```python
from build123d import *

# Parameters (mm, degrees)
SKETCH1_R                                 = 44.5
BOSS_EXTRUDE1_DEPTH                       = 24.13
SHELL1_T                                  = -5
CSK_FOR_0_FLAT_HEAD_MACHINE_SCREW_2_COUNT = 2
CSK_FOR_0_FLAT_HEAD_MACHINE_SCREW_2_PITCH = 69.412105808
CIRPATTERN1_COUNT                         = 8
FILLET1_R                                 = 10


with BuildPart() as part:
    # Sketch1 → Boss-Extrude1 (new, symmetric)
    with BuildSketch(Plane.XY):
        with Locations(Location((0, 0, 0), (0, 0, 180))):
            Circle(SKETCH1_R)
    extrude(amount=BOSS_EXTRUDE1_DEPTH, both=True)

    # Shell1
    shell1_openings = [part.faces().sort_by_distance(p)[0] for p in [
        (0, 0, 24.13),
    ]]
    offset(amount=SHELL1_T, openings=shell1_openings, kind=Kind.INTERSECTION)

    # Sketch5 → CSK for #0 Flat Head Machine Screw (100)1 (revolve, cut)
    with BuildSketch(Plane(origin=(-1.269301035, 41.980815558, 24.13), x_dir=(0, -1, 0), z_dir=(1, 0, 0))):
        Polygon((0, 0), (0, 3.07416509), (0.889, 2.54), (0.889, 0.5221717), (1.5113, 0), align=None)
    csk_for_0_flat_head_machine_screw_100 = revolve(axis=Axis((-1.269301035, 41.980815558, 30.48), (0, 0, -1)), mode=Mode.SUBTRACT)

    # CSK for _0 Flat Head Machine Screw _ 2: CSK for #0 Flat Head Machine Screw (100)1 ×2
    with Locations(*[Vector(0.9567328467758284, -0.2909677987341887, 0) * (i * CSK_FOR_0_FLAT_HEAD_MACHINE_SCREW_2_PITCH) for i in range(1, CSK_FOR_0_FLAT_HEAD_MACHINE_SCREW_2_COUNT)]):
        add(csk_for_0_flat_head_machine_screw_100, mode=Mode.SUBTRACT)

    # CirPattern1: CSK for #0 Flat Head Machine Screw (100)1 ×8 about axis
    cirpattern1_axis = Axis((0, 0, 0), (0, 0, 1))
    for i in range(1, CIRPATTERN1_COUNT):
        add(csk_for_0_flat_head_machine_screw_100.rotate(cirpattern1_axis, i * 360 / CIRPATTERN1_COUNT), mode=Mode.SUBTRACT)

    # CirPattern1 copy 1 sketch → CirPattern1 copy 1 (revolve, cut)
    with BuildSketch(Plane(origin=(30.656906272, 61.464315428, 24.13), x_dir=(0.7071067811865475, -0.7071067811865476, 0), z_dir=(0.7071067811865476, 0.7071067811865475, 0))):
        Polygon((0, 0), (0, 3.07416509), (0.889, 2.54), (0.889, 0.5221717), (1.5113, 0), align=None)
    revolve(axis=Axis((30.656906272, 61.464315428, 30.48), (0, 0, -1)), mode=Mode.SUBTRACT)

    # CirPattern1 copy 2 sketch → CirPattern1 copy 2 (revolve, cut)
    with BuildSketch(Plane(origin=(-21.784127925, 65.139540555, 24.13), x_dir=(1, 0, 0), z_dir=(0, 1, 0))):
        Polygon((0, 0), (0, 3.07416509), (0.889, 2.54), (0.889, 0.5221717), (1.5113, 0), align=None)
    revolve(axis=Axis((-21.784127925, 65.139540555, 30.48), (0, 0, -1)), mode=Mode.SUBTRACT)

    # CirPattern1 copy 3 sketch → CirPattern1 copy 3 (revolve, cut)
    with BuildSketch(Plane(origin=(-61.464315428, 30.656906272, 24.13), x_dir=(0.7071067811865476, 0.7071067811865475, 0), z_dir=(-0.7071067811865475, 0.7071067811865476, 0))):
        Polygon((0, 0), (0, 3.07416509), (0.889, 2.54), (0.889, 0.5221717), (1.5113, 0), align=None)
    revolve(axis=Axis((-61.464315428, 30.656906272, 30.48), (0, 0, -1)), mode=Mode.SUBTRACT)

    # CirPattern1 copy 4 sketch → CirPattern1 copy 4 (revolve, cut)
    with BuildSketch(Plane(origin=(-65.139540555, -21.784127925, 24.13), x_dir=(0, 1, 0), z_dir=(-1, 0, 0))):
        Polygon((0, 0), (0, 3.07416509), (0.889, 2.54), (0.889, 0.5221717), (1.5113, 0), align=None)
    revolve(axis=Axis((-65.139540555, -21.784127925, 30.48), (0, 0, -1)), mode=Mode.SUBTRACT)

    # CirPattern1 copy 5 sketch → CirPattern1 copy 5 (revolve, cut)
    with BuildSketch(Plane(origin=(-30.656906272, -61.464315428, 24.13), x_dir=(-0.7071067811865475, 0.7071067811865477, 0), z_dir=(-0.7071067811865477, -0.7071067811865475, 0))):
        Polygon((0, 0), (0, 3.07416509), (0.889, 2.54), (0.889, 0.5221717), (1.5113, 0), align=None)
    revolve(axis=Axis((-30.656906272, -61.464315428, 30.48), (0, 0, -1)), mode=Mode.SUBTRACT)

    # CirPattern1 copy 6 sketch → CirPattern1 copy 6 (revolve, cut)
    with BuildSketch(Plane(origin=(21.784127925, -65.139540555, 24.13), x_dir=(-1, 0, 0), z_dir=(0, -1, 0))):
        Polygon((0, 0), (0, 3.07416509), (0.889, 2.54), (0.889, 0.5221717), (1.5113, 0), align=None)
    revolve(axis=Axis((21.784127925, -65.139540555, 30.48), (0, 0, -1)), mode=Mode.SUBTRACT)

    # CirPattern1 copy 7 sketch → CirPattern1 copy 7 (revolve, cut)
    with BuildSketch(Plane(origin=(61.464315428, -30.656906272, 24.13), x_dir=(-0.7071067811865477, -0.7071067811865474, 0), z_dir=(0.7071067811865474, -0.7071067811865477, 0))):
        Polygon((0, 0), (0, 3.07416509), (0.889, 2.54), (0.889, 0.5221717), (1.5113, 0), align=None)
    revolve(axis=Axis((61.464315428, -30.656906272, 30.48), (0, 0, -1)), mode=Mode.SUBTRACT)

    # Fillet1
    fillet1_edges = [part.edges().sort_by_distance(p)[0] for p in [
        (44.5, 0, -24.13),
    ]]
    fillet(fillet1_edges, radius=FILLET1_R)


solid = part.part
```
CAD build for the part. Positions are in the model's coordinates, mm. A direction names the side the tool comes from. Coordinates: 2 decimals unless noted, no trailing zeros. Order: outer loops, then holes, each group sorted by start corner. A loop starts at its lowest first (then second) coordinate and runs counter-clockwise, first axis right, second up. Notation, with made-up numbers: (20, 37) - (54, 37) arc R19 ccw to (54, 72) - close; hole circle Ø7 at (-11, 22.25). An arc over 180 degrees is marked (long way). Answer in a Markdown table with one row per item.
1. Pull direction Y, two halves, no side cores. Call faces 3 (the face through (32.798, -30.075, 5.268)), 4 (the face through (40, -4, 24.13)), 5 (the face through (-37.676, -11.865, 2.803)): +Y half, -Y half, draft (parallel to the pull), parting line (faces both ways), or undercut.
Answer:
| item | result |
|---|---|
| face 3 | parting line |
| face 4 | draft |
| face 5 | undercut |
2. Flat gauge pins, fed straight in: P1, Ø1.1, axis at x = -41.98, y = -1.27, coming from the -Z side; P2, Ø2, axis at x = 28.79, y = 30.58, coming from the +Z side; P3, Ø3, axis at x = 1.27, y = -41.98, coming from the -Z side. Where does each tip first touch, or does it go through?
Answer:
| item | result |
|---|---|
| P1 | z = -21.32 |
| P2 | z = 23.7 |
| P3 | z = -22.13 |
3. Drill centre lines: L1, parallel to Y at x = 0, z = -2; L2, parallel to Z at x = 0, y = 7.5. Where is each one in solid material? Low to high. Write a range as from..to.
Answer:
| item | result |
|---|---|
| L1 | -44.5..-39.5, 39.5..44.5 |
| L2 | -24.13..-19.13 |
4. Slice it at A-A, the plane z = 4. List the corners of the cut face in (x, y), then the cut area to 3 significant figures.
Answer:
| item | result |
|---|---|
| outline | circle Ø89 at (0, 0); hole circle Ø79 at (0, 0) |
| area | 1,320 mm² |
5. 3-axis set-ups, long thin cutter, end or side, ignore diameter. For faces 1 (the face through (0, 0, -24.13)), 2 (the face through (1, -1, -19.13)): which of +Z, -Z, +X, -X, +Y, -Y reach the whole face in a straight line?
Answer:
| item | result |
|---|---|
| face 1 | -Z, +X, -X, +Y, -Y |
| face 2 | +Z |
